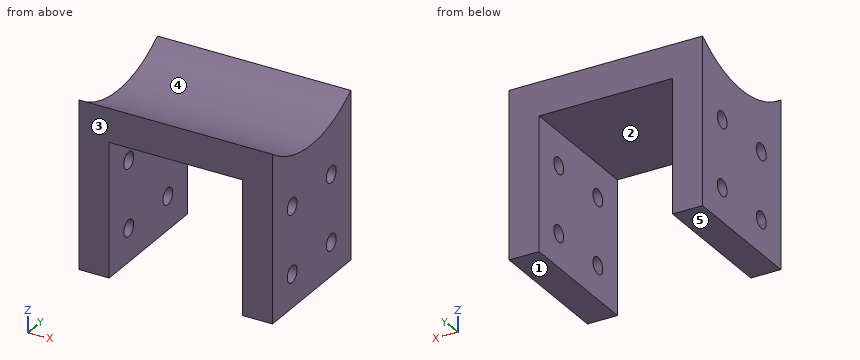
```python
from build123d import *

# Parameters (mm, degrees)
BOSS_EXTRUDE1_DEPTH     = 40
SKETCH4_R               = 2.5
CUT_EXTRUDE1_DEPTH      = 50
CUT_EXTRUDE1_DEPTH_BACK = 10
CUT_EXTRUDE2_DEPTH      = 59


with BuildPart() as part:
    # Sketch1 → Boss-Extrude1 (new body)
    with BuildSketch(Plane(origin=(0, 0, 0), x_dir=(1, 0, 0), z_dir=(0, 1, 0))):
        Polygon((0, 0), (58, 0), (58, 50), (49, 50), (49, 10), (9, 10), (9, 50), (0, 50), align=None)
    extrude(amount=BOSS_EXTRUDE1_DEPTH)

    # Sketch4 → Cut-Extrude1 (cut, two sides)
    with BuildSketch(Plane.ZY.offset(-49)) as cut_extrude1_sk:
        with BuildLine():
            ThreePointArc((-42.5, 10), (-41.767766953, 8.232233047), (-40, 7.5))
            Line((-40, 7.5), (-40, 10))
            Line((-40, 10), (-42.5, 10))
        make_face()
        with BuildLine():
            Line((-40, 10), (-40, 7.5))
            ThreePointArc((-40, 7.5), (-38.232233047, 8.232233047), (-37.5, 10))
            ThreePointArc((-37.5, 10), (-40, 12.5), (-42.5, 10))
            Line((-42.5, 10), (-40, 10))
        make_face()
        with Locations((-20, 10)):
            Circle(SKETCH4_R)
        with Locations((-40, 30)):
            Circle(SKETCH4_R)
        with Locations((-20, 30)):
            Circle(SKETCH4_R)
    extrude(amount=CUT_EXTRUDE1_DEPTH, mode=Mode.SUBTRACT)
    extrude(cut_extrude1_sk.sketch, amount=-CUT_EXTRUDE1_DEPTH_BACK, mode=Mode.SUBTRACT)

    # Sketch5 → Cut-Extrude2 (cut, through all)
    with BuildSketch(Plane(origin=(58, 0, 0), x_dir=(0, 0, -1), z_dir=(1, 0, 0))):
        with BuildLine():
            Line((0, 40), (0, 0))
            ThreePointArc((0, 0), (6.50454583, 20), (0, 40))
        make_face()
    extrude(amount=-CUT_EXTRUDE2_DEPTH, mode=Mode.SUBTRACT)


solid = part.part
```
Here's how the part is built. I have some questions about the finished solid (model axes, mm). Face numbers are marked on the shaded views. A direction names the side the tool comes from. Give positions to 0.01 mm unless a question says otherwise; leave off trailing zeros. Write each loop counter-clockwise with the first axis right and the second up, starting at its lowest first coordinate (ties: lowest second). Pieces come first, ordered by that corner, then holes. Notation, with made-up numbers: (-4.75, -3) -> (4.25, -3) arc R14 cw to (4.25, 12) -> close; hole circle Ø2 at (-29.5, -7.5). An arc over 180 degrees is marked (long way). Use one line per item in the form item = value.
1) Suppose I cut it at B-B (y = 11). Please give me the cut outline in (x, z), and give its area (3 significant figures).
Verdict:
outline = (0, -50) -> (9, -50) -> (9, -42.29) -> (0, -42.29) -> close; (0, -37.71) -> (9, -37.71) -> (9, -22.29) -> (0, -22.29) -> close; (0, -17.71) -> (9, -17.71) -> (9, -10) -> (49, -10) -> (49, -17.71) -> (58, -17.71) -> (58, -5.29) -> (0, -5.29) -> close; (49, -50) -> (58, -50) -> (58, -42.29) -> (49, -42.29) -> close; (49, -37.71) -> (58, -37.71) -> (58, -22.29) -> (49, -22.29) -> close
area = 828 mm2
2) Suppose I cut it at C-C (x = 35). Please give me the cut outline in (y, z).
Verdict:
outline = (0, -10) -> (40, -10) -> (40, 0) arc R34 cw to (0, 0) -> close
3) Suppose I cut it at D-D (y = 30). Please give me the cut outline in (x, z), and give its area (3 significant figures).
Verdict:
outline = (0, -50) -> (9, -50) -> (9, -42.5) -> (0, -42.5) -> close; (0, -37.5) -> (9, -37.5) -> (9, -22.5) -> (0, -22.5) -> close; (0, -17.5) -> (9, -17.5) -> (9, -10) -> (49, -10) -> (49, -17.5) -> (58, -17.5) -> (58, -5) -> (0, -5) -> close; (49, -50) -> (58, -50) -> (58, -42.5) -> (49, -42.5) -> close; (49, -37.5) -> (58, -37.5) -> (58, -22.5) -> (49, -22.5) -> close
area = 830 mm2
4) I'm going to push flat-ended pins straight in: pin 1 (1 mm diameter, centred on y = 36, z = -21.5, fed in from -X); pin 2 (12 mm diameter, centred on x = 35.5, y = 21, fed in from +Z); pin 3 (3 mm diameter, centred on x = 36, y = 8.5, fed in from -Z); pin 4 (3 mm diameter, centred on x = 26.5, y = 28.5, fed in from +Z). Where does each tip first touch, or does it pass through?
Verdict:
pin_1 = 0
pin_2 = -5.78
pin_3 = -10
pin_4 = -5
5) We'd pull the mould along Y, two halves only. Please class the marked faces 3, 4 and 5: +Y half, -Y half, draft (parallel to the pull), parting line (faces both ways), or undercut.
Verdict:
face_3 = -Y half
face_4 = undercut
face_5 = draft
6) If I drill on L1, parallel to Y at x = 52.75, z = -20; L2, parallel to X at y = 20, z = -46.5; L3, parallel to Z at x = 4.5, y = 30, over which ranges is the centre line in solid material (lowest first)? Write a range as [from, to].
Verdict:
L1 = [0, 7.5], [12.5, 27.5], [32.5, 40]
L2 = [0, 9], [49, 58]
L3 = [-50, -42.5], [-37.5, -22.5], [-17.5, -5]
7) Suppose I cut it at A-A (z = -20). Please give me the cut outline in (x, y).
Verdict:
outline = (0, 0) -> (9, 0) -> (9, 7.5) -> (0, 7.5) -> close; (0, 12.5) -> (9, 12.5) -> (9, 27.5) -> (0, 27.5) -> close; (0, 32.5) -> (9, 32.5) -> (9, 40) -> (0, 40) -> close; (49, 0) -> (58, 0) -> (58, 7.5) -> (49, 7.5) -> close; (49, 12.5) -> (58, 12.5) -> (58, 27.5) -> (49, 27.5) -> close; (49, 32.5) -> (58, 32.5) -> (58, 40) -> (49, 40) -> close
8) On a 3-axis mill with a long thin cutter (end or side, diameter ignored), from which of +Z, -Z, +X, -X, +Y, -Y can I reach the whole of each face in a straight line? I mean the marked faces 1 and 2. Say none if no direction works.
Verdict:
face_1 = -Z, +X, -X, +Y, -Y
face_2 = -Z, +Y, -Y
